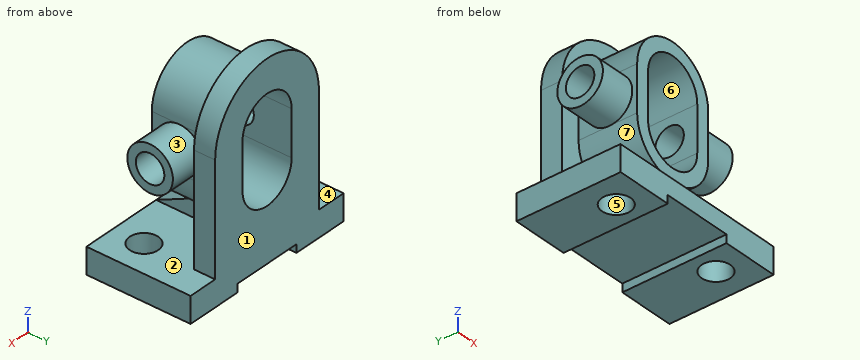
```python
from build123d import *

# Parameters (mm, degrees)
SKETCH_1_W           = 224
SKETCH_1_H           = 128
SKETCH_1_R           = 17.5
EXTRUDE_1_DEPTH      = 32
SKETCH_2_W           = 86
SKETCH_2_H           = 20
CUT_EXTRUDE_1_DEPTH  = 145
EXTRUDE_2_DEPTH      = 26
EXTRUDE_3_DEPTH      = 72
CUT_EXTRUDE_2_DEPTH  = 131
SKETCH_6_R           = 28
EXTRUDE_5_DEPTH      = 43
EXTRUDE_START        = 43
SKETCH_7_R           = 28
EXTRUDE_6_DEPTH      = 43
SKETCH_8_R           = 17.5
CUT_EXTRUDE_3_DEPTH  = 241
EXTRUDE_7_DEPTH      = 10
EXTRUDE_7_DEPTH_BACK = 10


with BuildPart() as part:
    # 草图1 → 凸台-拉伸1 (new body)
    with BuildSketch(Plane.XY):
        Rectangle(SKETCH_1_W, SKETCH_1_H)
        with Locations((73, -26)):
            Circle(SKETCH_1_R, mode=Mode.SUBTRACT)
        with Locations(Location((-73, -26, 0), (0, 0, 180))):
            Circle(SKETCH_1_R, mode=Mode.SUBTRACT)
    extrude(amount=EXTRUDE_1_DEPTH)

    # 草图2 → 切除-拉伸1 (cut)
    with BuildSketch(Plane.XZ.offset(64)):
        Rectangle(SKETCH_2_W, SKETCH_2_H)
    extrude(amount=-CUT_EXTRUDE_1_DEPTH, mode=Mode.SUBTRACT)

    # 草图3 → 凸台-拉伸2 (add)
    with BuildSketch(Plane(origin=(0, 64, 0), x_dir=(1, 0, 0), z_dir=(0, 1, 0))):
        with BuildLine():
            Line((76, -168), (76, -32))
            Line((76, -32), (-76, -32))
            Line((-76, -32), (-76, -168))
            ThreePointArc((-76, -168), (0, -244), (76, -168))
        make_face()
    extrude(amount=-EXTRUDE_2_DEPTH)

    # 草图4 → 凸台-拉伸3 (add)
    with BuildSketch(Plane.XZ.offset(-38)):
        with BuildLine():
            Line((-52, 168), (-52, 112))
            ThreePointArc((-52, 112), (0, 60), (52, 112))
            Line((52, 112), (52, 168))
            ThreePointArc((52, 168), (0, 220), (-52, 168))
        make_face()
    extrude(amount=EXTRUDE_3_DEPTH)

    # 草图5 → 切除-拉伸2 (cut)
    with BuildSketch(Plane.XZ.offset(34)):
        with BuildLine():
            Line((-36, 168), (-36, 112))
            ThreePointArc((-36, 112), (0, 76), (36, 112))
            Line((36, 112), (36, 168))
            ThreePointArc((36, 168), (0, 204), (-36, 168))
        make_face()
    extrude(amount=-CUT_EXTRUDE_2_DEPTH, mode=Mode.SUBTRACT)

    # 草图6 → 凸台-拉伸5 (add)
    with BuildSketch(Plane.ZY.offset(52)):
        with Locations(Location((140, 0, 0), (0, 0, 180))):
            Circle(SKETCH_6_R)
    extrude(amount=EXTRUDE_5_DEPTH)

    # 草图7 → 凸台-拉伸6 (add)
    with BuildSketch(Plane(origin=(52, 0, 0), x_dir=(0, 0, -1), z_dir=(1, 0, 0)).offset(EXTRUDE_START)):
        with Locations((-140, 0)):
            Circle(SKETCH_7_R)
    extrude(amount=-EXTRUDE_6_DEPTH)

    # 草图8 → 切除-拉伸3 (cut)
    with BuildSketch(Plane.ZY.offset(95)):
        with Locations(Location((140, 0, 0), (0, 0, 90))):
            Circle(SKETCH_8_R)
    extrude(amount=-CUT_EXTRUDE_3_DEPTH, mode=Mode.SUBTRACT)

    # 草图9 → 凸台-拉伸7 (add, two sides: drawn at the far end of the back side and taken through both)
    with BuildSketch(Plane(origin=(0, 0, 0), x_dir=(0, 0, -1), z_dir=(1, 0, 0)).offset(-EXTRUDE_7_DEPTH_BACK)):
        Polygon((-52, -22), (-67.637033122, -22), (-67.637033122, 38), (-32, 38), (-32, -64), align=None)
    extrude(amount=EXTRUDE_7_DEPTH + EXTRUDE_7_DEPTH_BACK)


solid = part.part
```
Part model, mm, in its own coordinate system. Face numbers are marked on the shaded views. A direction names the side the tool comes from. Round coordinates to 2 decimals unless told otherwise and drop trailing zeros. Loops run counter-clockwise (first coordinate to the right, second up) from the corner with the lowest first, then second, coordinate; pieces in that order, holes last.
Item 1: Cut at A-A, the plane x = 0. Give the cut face in (y, z).
Item 2: Cut at C-C, the plane y = 50. Give the cut face in (x, z), then the cut area to 3 significant figures.
Item 3: Cut at B-B, the plane z = 140. Give the cut face in (x, y).
Item 4: Drop flat-ended pins along their axis: P1, Ø1, axis at y = 39, z = 46.5, coming from the -X side; P2, Ø11.5, axis at y = 15, z = 152, coming from the +X side; P3, Ø2.5, axis at x = 3.5, z = 55.5, coming from the -Y side. Give the stop position or say it passes through.
Item 5: 3-axis set-ups, long thin cutter, end or side, ignore diameter. For the marked faces 4, 5, 6 and 7: which of +Z, -Z, +X, -X, +Y, -Y reach the whole face in a straight line?
Item 6: Drill centre lines: line 1 (Y direction, x = -73, z = 12); line 2 (Y direction, x = 53, z = 140); line 3 (X direction, y = 13.5, z = 166). Where is each one in solid material? Low to high.
Item 7: Mould opens along Y. For the marked faces 1, 2 and 3 say: +Y half, -Y half, draft (parallel to the pull), parting line (faces both ways), or undercut.
Item 8: Cut at D-D, the plane z = 115. Give the cut face in (x, y).
A:
1. outline: (-64, 10) - (64, 10) - (64, 76) - (-34, 76) - (-34, 60) - (-22, 60) - (-22, 52) - (-64, 32) - close; (-34, 204) - (64, 204) - (64, 244) - (38, 244) - (38, 220) - (-34, 220) - close
2. outline: (-112, 0) - (-43, 0) - (-43, 10) - (43, 10) - (43, 0) - (112, 0) - (112, 32) - (76, 32) - (76, 168) arc R76 ccw to (-76, 168) - (-76, 32) - (-112, 32) - close; hole (-36, 112) arc R36 ccw to (36, 112) - (36, 168) arc R36 ccw to (-36, 168) - close
2. area: 27,900 mm2
3. outline: (-95, -28) - (-52, -28) - (-52, -34) - (-36, -34) - (-36, -17.5) - (-95, -17.5) - close; (-95, 17.5) - (-36, 17.5) - (-36, 64) - (-76, 64) - (-76, 38) - (-52, 38) - (-52, 28) - (-95, 28) - close; (36, -34) - (52, -34) - (52, -28) - (95, -28) - (95, -17.5) - (36, -17.5) - close; (36, 17.5) - (95, 17.5) - (95, 28) - (52, 28) - (52, 38) - (76, 38) - (76, 64) - (36, 64) - close
4. P1: stops at x = -76
4. P2: stops at x = 95
4. P3: stops at y = -22
5. face 4: -X, -Y
5. face 5: -Z
5. face 6: +Y, -Y
5. face 7: -Y
6. line 1: y = -64 to -43.5, -8.5 to 64
6. line 2: y = -28 to -17.5, 17.5 to 28, 38 to 64
6. line 3: x = -52 to -36, 36 to 52
7. face 1: +Y half
7. face 2: draft
7. face 3: undercut
8. outline: (-95, -12.61) - (-52, -12.61) - (-52, -34) - (-36, -34) - (-36, 64) - (-76, 64) - (-76, 38) - (-52, 38) - (-52, 12.61) - (-95, 12.61) - close; (36, -34) - (52, -34) - (52, -12.61) - (95, -12.61) - (95, 12.61) - (52, 12.61) - (52, 38) - (76, 38) - (76, 64) - (36, 64) - close
